from build123d import *

# Parameters (mm, degrees)
F0_R     = 75
F1_DEPTH = 15
F2_R     = 57.5
F3_DEPTH = 25
F4_R     = 3.175
F4_R_2   = 1.5875
F5_DEPTH = 40.001


with BuildPart() as f1:
    # F0 (on Front) → F1 (new body)
    with BuildSketch(Plane.XZ):
        Circle(F0_R)
    extrude(amount=F1_DEPTH)

    # F2 (on face) → F3 (join)
    with BuildSketch(Plane(origin=(0, 0, 0), x_dir=(-1, 0, 0), z_dir=(0, 1, 0))):
        Circle(F2_R)
    extrude(amount=F3_DEPTH)

    # F4 (on face) → F5 (cut, through all)
    with BuildSketch(Plane.XZ.offset(15)):
        Circle(F4_R)
        with Locations((-40, 0)):
            Circle(F4_R_2)
    extrude(amount=-F5_DEPTH, mode=Mode.SUBTRACT)


solid = f1.part
Geometry: final body of the model. Coordinates: model frame, mm. A direction names the side the tool comes from. Give positions to 0.01 mm unless a question says otherwise; leave off trailing zeros. Write each loop counter-clockwise with the first axis right and the second up, starting at its lowest first coordinate (ties: lowest second). Pieces come first, ordered by that corner, then holes. Notation, with made-up numbers: (-24.75, 7.25) - (21.25, 7.25) arc R22 ccw to (21.25, 38.25) - close; hole circle Ø5 at (-3, -12.75). An arc over 180 degrees is marked (long way). Return JSON: item names as keys, results as strings. Group by question number.
1) Line query: line 1 (Z direction, x = 0, y = 9) (3 decimals); line 2 (Z direction, x = -40, y = -3); line 3 (Y direction, x = 40, z = 50). Output: solid intervals per line, ascending.
2) Section B-B on y = 21.5. State how many separate pieces and enclosed holes the cut face has, plus the area to 3 significant figures.
3) Section C-C on z = -5.5. Return the cut outline in (x, y), plus the area to 3 significant figures.
4) Section A-A on x = 0. Return the cut outline in (y, z) (3 decimals).
5) Section D-D on x = -52. Return the cut outline in (y, z).
6) First-contact query: P1, Ø12, axis at y = 18.5, z = 55.5, coming from the -X side; P2, Ø5, axis at x = -15, y = 16, coming from the -Z side; P3, Ø12, axis at y = 8.5, z = -46.5, coming from the -X side. Flat tips, straight axial feed; report the tip coordinate or a pass-through.
7) Set-up query: faces 1 (the flat face through (-12, 25, 1)), 2 (the cylindrical face through (12.465, 12.325, -56.133)). Return all of +Z, -Z, +X, -X, +Y, -Y with unobstructed straight access to the full face (end or side cutting, diameter ignored); none if empty.
Filled in:
{
 "1": {"line 1": "z = -57.5 to -3.175, 3.175 to 57.5", "line 2": "z = -63.44 to -1.59, 1.59 to 63.44", "line 3": "y = -15 to 0"},
 "2": {"separate pieces": "1", "enclosed holes": "2", "area": "10,300 mm^2"},
 "3": {"outline": "(-74.8, -15) - (74.8, -15) - (74.8, 0) - (57.24, 0) - (57.24, 25) - (-57.24, 25) - (-57.24, 0) - (-74.8, 0) - close", "area": "5,110 mm^2"},
 "4": {"outline": "(-15, -75) - (0, -75) - (0, -57.5) - (25, -57.5) - (25, -3.175) - (-15, -3.175) - close; (-15, 3.175) - (25, 3.175) - (25, 57.5) - (0, 57.5) - (0, 75) - (-15, 75) - close"},
 "5": {"outline": "(-15, -54.05) - (0, -54.05) - (0, -24.54) - (25, -24.54) - (25, 24.54) - (0, 24.54) - (0, 54.05) - (-15, 54.05) - close"},
 "6": {"P1": "stops at x = -29.26", "P2": "stops at z = -56.12", "P3": "stops at x = -40.82"},
 "7": {"face 1": "+Z, -Z, +X, -X, +Y", "face 2": "+Y"}
}
